```python
from build123d import *

# Parameters (mm, degrees)
SKETCH1_W           = 34
SKETCH1_H           = 26.5
SKETCH1_R           = 1.5
BOSS_EXTRUDE1_DEPTH = 1.5
SKETCH2_W           = 19.764821035
SKETCH2_H           = 13.28137913
BOSS_EXTRUDE2_DEPTH = 15.5
SKETCH3_W           = 4.088439113
SKETCH3_H           = 14.781279869
BOSS_EXTRUDE3_DEPTH = 10


with BuildPart() as part:
    # Sketch1 → Boss-Extrude1 (new body)
    with BuildSketch(Plane.XY):
        with Locations((17, 13.25)):
            Rectangle(SKETCH1_W, SKETCH1_H)
        with Locations((2, 24.5)):
            Circle(SKETCH1_R, mode=Mode.SUBTRACT)
        with Locations((32, 24.5)):
            Circle(SKETCH1_R, mode=Mode.SUBTRACT)
        with Locations((2, 2)):
            Circle(SKETCH1_R, mode=Mode.SUBTRACT)
        with Locations((32, 2)):
            Circle(SKETCH1_R, mode=Mode.SUBTRACT)
    extrude(amount=BOSS_EXTRUDE1_DEPTH)

    # Sketch2 → Boss-Extrude2 (add)
    with BuildSketch(Plane.XY.offset(1.5)):
        with Locations((14.883204602, 12.306514051)):
            Rectangle(SKETCH2_W, SKETCH2_H)
    extrude(amount=BOSS_EXTRUDE2_DEPTH)

    # Sketch3 → Boss-Extrude3 (add)
    with BuildSketch(Plane.XY.offset(1.5)):
        with Locations((27.511401151, 13.177424158)):
            Rectangle(SKETCH3_W, SKETCH3_H)
    extrude(amount=BOSS_EXTRUDE3_DEPTH)


solid = part.part
```
The model under review builds one solid part; all positions refer to its coordinate system, in mm. A direction names the side the tool comes from. Round coordinates to 2 decimals unless told otherwise and drop trailing zeros. Loops run counter-clockwise (first coordinate to the right, second up) from the corner with the lowest first, then second, coordinate; pieces in that order, holes last. Notation, with made-up numbers: M 7,-16.5 L 51,-16.5 A28 cw 51,12.5 Z; hole C 37.25,77 d4. An arc over 180 degrees is marked long. Write item = value, one per line.
Item 1: Take a section at D-D on x = 18.5. Write out the cut boundary in (y, z), then the cut area to 3 significant figures.
Return value:
outline = M 0,0 L 26.5,0 L 26.5,1.5 L 18.95,1.5 L 18.95,17 L 5.67,17 L 5.67,1.5 L 0,1.5 Z
area = 246 mm2
Item 2: The part is to be moulded in two halves that separate along Y. For faces 1 (the flat face through (17, 13, 0)), 2 (the cylindrical face through (30.89, 25.51, 0.74)), 3 (the cylindrical face through (2, 26, 1)), 4 (the flat face through (27, 5.787, 6)), say which applies: released by +Y, released by -Y, zero draft, split by the parting line, or undercut.
Return value:
face_1 = zero draft
face_2 = undercut
face_3 = undercut
face_4 = released by -Y
Item 3: Take a section at A-A on y = 24.5. Write out the cut boundary in (x, z), then the cut area to 3 significant figures.
Return value:
outline = M 0,0 L 0.5,0 L 0.5,1.5 L 0,1.5 Z; M 3.5,0 L 30.5,0 L 30.5,1.5 L 3.5,1.5 Z; M 33.5,0 L 34,0 L 34,1.5 L 33.5,1.5 Z
area = 42.0 mm2
Item 4: Take a section at B-B on z = 9.25. Write out the cut boundary in (x, y), then the cut area to 3 significant figures.
Return value:
outline = M 5,5.67 L 24.77,5.67 L 24.77,18.95 L 5,18.95 Z; M 25.47,5.79 L 29.56,5.79 L 29.56,20.57 L 25.47,20.57 Z
area = 323 mm2
Item 5: Machinability: for faces 5 (the flat face through (5.001, 12, 9)), 6 (the flat face through (27, 13, 11.5)), 7 (the flat face through (15, 18.947, 9)), 8 (the flat face through (27, 20.568, 6)), 9 (the flat face through (24.766, 12, 9)), which of the approach directions +Z, -Z, +X, -X, +Y, -Y give a long, thin tool a straight path to every point of the face, cutting with its end or side? Answer none if there is none.
Return value:
face_5 = +Z, -X, +Y, -Y
face_6 = +Z, +X, +Y, -Y
face_7 = +Z, -X, +Y
face_8 = +Z, +X, -X, +Y
face_9 = +Z, +Y, -Y
Item 6: Insertion check: P1, Ø1.8, axis at x = 32, y = 2, coming from the -Z side; P2, Ø3, axis at x = 4.5, z = 7, coming from the +Y side; P3, Ø3.5, axis at x = 27.5, z = 5, coming from the -Y side; P4, Ø5, axis at x = 22, y = 5.5, coming from the -Z side. Each pin has a flat end and moves straight along its axis. Give the tip position at first contact, or say it passes through.
Return value:
P1 = through
P2 = 18.95
P3 = 5.79
P4 = 0
Item 7: For line 1 (Y direction, x = 2, z = 1.1); line 2 (Z direction, x = 5, y = 24); line 3 (Y direction, x = 20, z = 4.5), list the stretches that pass through material, from the lowest coordinate up. Write a range as [from, to].
Return value:
line_1 = [0, 0.5], [3.5, 23], [26, 26.5]
line_2 = [0, 1.5]
line_3 = [5.67, 18.95]
Item 8: Take a section at C-C on x = 2. Write out the cut boundary in (y, z).
Return value:
outline = M 0,0 L 0.5,0 L 0.5,1.5 L 0,1.5 Z; M 3.5,0 L 23,0 L 23,1.5 L 3.5,1.5 Z; M 26,0 L 26.5,0 L 26.5,1.5 L 26,1.5 Z
